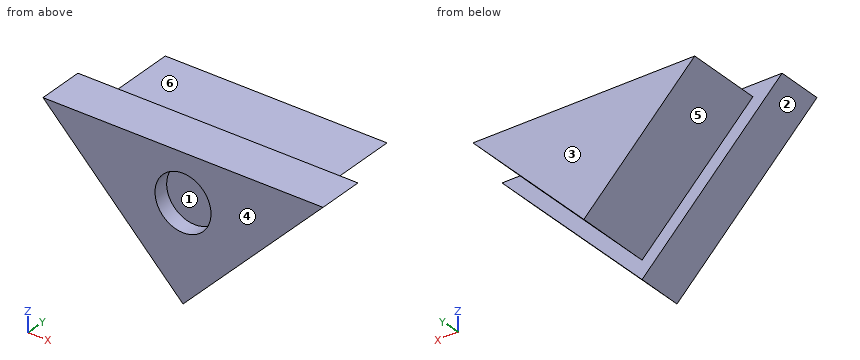
from build123d import *

# Parameters (mm, degrees)
BOSS_EXTRUDE1_DEPTH = 3
BOSS_EXTRUDE2_DEPTH = 5
SKETCH3_R           = 1.8
CUT_EXTRUDE1_DEPTH  = 1


with BuildPart() as part:
    # Sketch1 → Boss-Extrude1 (new body)
    with BuildSketch(Plane(origin=(0, 0, 0), x_dir=(1, 0, 0), z_dir=(0, 1, 0))):
        Polygon((8.983252998, -8.397111121), (-9.016747002, -8.397111121), (-0.016747002, 0.756293591), align=None)
    extrude(amount=BOSS_EXTRUDE1_DEPTH)

    # Sketch2 → Boss-Extrude2 (add)
    with BuildSketch(Plane(origin=(0, 3, 0), x_dir=(1, 0, 0), z_dir=(0, 1, 0))):
        Polygon((7.109021951, -7.663380877), (-0.015978049, -0.416935476), (-7.141084887, -7.663380877), align=None)
    extrude(amount=BOSS_EXTRUDE2_DEPTH)

    # Sketch3 → Cut-Extrude1 (cut)
    with BuildSketch(Plane.XZ):
        with Locations(Location((-0.016747002, 5.345976217, 0), (0, 0, 270))):
            Circle(SKETCH3_R)
    extrude(amount=-CUT_EXTRUDE1_DEPTH, mode=Mode.SUBTRACT)


solid = part.part
Work out the finished part from the listing and answer in its coordinate system (mm). Face numbers are marked on the shaded views. A direction names the side the tool comes from. Give positions to 0.01 mm unless a question says otherwise; leave off trailing zeros. Loops run counter-clockwise (first coordinate to the right, second up) from the corner with the lowest first, then second, coordinate; pieces in that order, holes last. Notation, with made-up numbers: (-37, -26) -> (-25, -26) arc R24 cw to (-25, 4) -> close; hole circle Ø9 at (32, -7.5). An arc over 180 degrees is marked (long way). Use a Markdown table: item, result. Add a question column.
1) The part is cut by section C-C, the plane y = 2.25. Determine the outline of the cut face in (x, z).
2) Each of these flat-tipped pins is pushed along its axis until it touches: P1, Ø3, axis at x = -0.02, z = 5.35, coming from the -Y side; P2, Ø1.5, axis at y = 7, z = 3, coming from the +X side; P3, Ø4, axis at y = 4, z = 6.5, coming from the +X side. Where does it stop, or does it pass through?
3) For a pull along Z with two mould halves and no side action, classify the marked faces 1, 2 and 3 as +Z half, -Z half, draft (parallel to the pull), parting line (faces both ways), or undercut.
4) The part is cut by section B-B, the plane x = -1.25. Determine the outline of the cut face in (y, z).
5) Consider line 1 along Y through (x, z) = (-0.25, 7); line 2 along Y through (x, z) = (6.5, 7); line 3 along Z through (x, y) = (1.5, 4.75). Determine where each line is inside the solid, lowest interval first.
6) The part is cut by section D-D, the plane x = 3.5. Determine the outline of the cut face in (y, z), plus the area to 3 significant figures.
7) Which of the six approach directions +Z, -Z, +X, -X, +Y, -Y give full straight-line access (tool end or side, diameter ignored) to the marked faces 4, 5 and 6?
8) The part is cut by section A-A, the plane z = 3.75. Determine the outline of the cut face in (x, y).
Reported:
| question | item | result |
|---|---|---|
| 1 | outline | (-9.02, 8.4) -> (-0.02, -0.76) -> (8.98, 8.4) -> close |
| 2 | P1 | stops at y = 1 |
| 2 | P2 | stops at x = 3.26 |
| 2 | P3 | stops at x = 8.82 |
| 3 | face 1 | undercut |
| 3 | face 2 | -Z half |
| 3 | face 3 | draft |
| 4 | outline | (0, 0.5) -> (3, 0.5) -> (3, 1.67) -> (8, 1.67) -> (8, 7.66) -> (3, 7.66) -> (3, 8.4) -> (0, 8.4) -> (0, 6.66) -> (1, 6.66) -> (1, 4.03) -> (0, 4.03) -> close |
| 5 | line 1 | y = 1 to 8 |
| 5 | line 2 | y = 0 to 3 |
| 5 | line 3 | z = 1.96 to 7.66 |
| 6 | outline | (0, 2.82) -> (3, 2.82) -> (3, 3.99) -> (8, 3.99) -> (8, 7.66) -> (3, 7.66) -> (3, 8.4) -> (0, 8.4) -> close |
| 6 | area | 35.1 mm^2 |
| 7 | face 4 | +Z, -Z, +X, -X, -Y |
| 7 | face 5 | -Z, -X, +Y |
| 7 | face 6 | +Z, +X, -X, +Y |
| 8 | outline | (-4.45, 0) -> (-0.85, 0) -> (-0.85, 1) -> (0.82, 1) -> (0.82, 0) -> (4.41, 0) -> (4.41, 3) -> (3.26, 3) -> (3.26, 8) -> (-3.29, 8) -> (-3.29, 3) -> (-4.45, 3) -> close |
